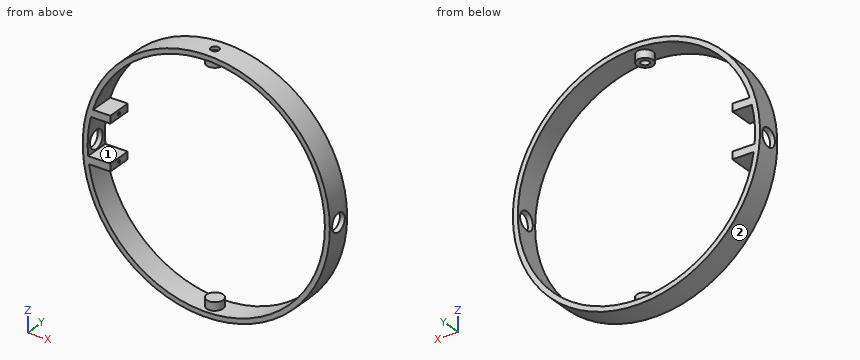
from build123d import *

# Parameters (mm, degrees)
SKETCH1_R               = 75
SKETCH1_R_2             = 72
BOSS_EXTRUDE1_DEPTH     = 15
SKETCH2_R               = 5.5
CUT_EXTRUDE1_DEPTH      = 76
CUT_EXTRUDE1_DEPTH_BACK = 76
BOSS_EXTRUDE2_START     = -6
SKETCH3_R               = 5
BOSS_EXTRUDE2_DEPTH     = 7
SKETCH4_W               = 11.8125703
SKETCH4_H               = 4.5
SKETCH4_W_2             = 13.541131856
BOSS_EXTRUDE3_DEPTH     = 15
SKETCH5_R               = 0.9
CUT_EXTRUDE2_DEPTH      = 8
SKETCH6_R               = 2.45
CUT_EXTRUDE3_DEPTH      = 4
SKETCH7_R               = 1.25
CUT_EXTRUDE4_DEPTH      = 4
SKETCH8_R               = 2.5
CUT_EXTRUDE5_DEPTH      = 4


with BuildPart() as part:
    # Sketch1 → Boss-Extrude1 (new body)
    with BuildSketch(Plane(origin=(0, 0, 0), x_dir=(1, 0, 0), z_dir=(0, 1, 0))):
        Circle(SKETCH1_R)
        Circle(SKETCH1_R_2, mode=Mode.SUBTRACT)
    extrude(amount=BOSS_EXTRUDE1_DEPTH)

    # Sketch2 → Cut-Extrude1 (cut, two sides)
    with BuildSketch(Plane(origin=(0, 0, 0), x_dir=(0, 0, -1), z_dir=(1, 0, 0))) as cut_extrude1_sk:
        with Locations((0, 7.5)):
            Circle(SKETCH2_R)
    extrude(amount=CUT_EXTRUDE1_DEPTH, mode=Mode.SUBTRACT)
    extrude(cut_extrude1_sk.sketch, amount=-CUT_EXTRUDE1_DEPTH_BACK, mode=Mode.SUBTRACT)

    # Sketch3 → Boss-Extrude2 (add)
    with BuildSketch(Plane.XY.offset(73).offset(BOSS_EXTRUDE2_START)):
        with Locations((0, 7.5)):
            Circle(SKETCH3_R)
    boss_extrude2 = extrude(amount=BOSS_EXTRUDE2_DEPTH)

    # Mirror1: Boss-Extrude2 across plane
    add(boss_extrude2.mirror(Plane.XY))

    # Sketch4 → Boss-Extrude3 (add)
    with BuildSketch(Plane(origin=(0, 15, 0), x_dir=(1, 0, 0), z_dir=(0, 1, 0))):
        with Locations((-64.10628515, -19.05)):
            Rectangle(SKETCH4_W, SKETCH4_H)
        with Locations((-64.970565928, 8.35)):
            Rectangle(SKETCH4_W_2, SKETCH4_H)
    extrude(amount=-BOSS_EXTRUDE3_DEPTH)

    # Sketch5 → Cut-Extrude2 (cut)
    with BuildSketch(Plane(origin=(-58.2, 0, 0), x_dir=(0, 0, -1), z_dir=(1, 0, 0))):
        with Locations((8.3, 7.5)):
            Circle(SKETCH5_R)
        with Locations((-19, 7.5)):
            Circle(SKETCH5_R)
    extrude(amount=-CUT_EXTRUDE2_DEPTH, mode=Mode.SUBTRACT)

    # Sketch6 → Cut-Extrude3 (cut)
    with BuildSketch(Plane(origin=(0, 0, 67), x_dir=(-1, 0, 0), z_dir=(0, 0, -1))):
        with Locations((0, 7.5)):
            Circle(SKETCH6_R)
    extrude(amount=-CUT_EXTRUDE3_DEPTH, mode=Mode.SUBTRACT)

    # Sketch7 → Cut-Extrude4 (cut)
    with BuildSketch(Plane(origin=(0, 0, 71), x_dir=(-1, 0, 0), z_dir=(0, 0, -1))):
        with Locations((0, 7.5)):
            Circle(SKETCH7_R)
    extrude(amount=-CUT_EXTRUDE4_DEPTH, mode=Mode.SUBTRACT)

    # Sketch8 → Cut-Extrude5 (cut)
    with BuildSketch(Plane(origin=(0, 0, 73), x_dir=(-1, 0, 0), z_dir=(0, 0, -1))):
        with Locations((0, 7.5)):
            Circle(SKETCH8_R)
    extrude(amount=-CUT_EXTRUDE5_DEPTH, mode=Mode.SUBTRACT)


solid = part.part
Source: CAD feature listing. Evaluate the final solid. Frame: model axes, mm. Face numbers are marked on the shaded views. Round coordinates to 2 decimals unless told otherwise and drop trailing zeros. Write each loop counter-clockwise with the first axis right and the second up, starting at its lowest first coordinate (ties: lowest second). Pieces come first, ordered by that corner, then holes. Notation, with made-up numbers: M -38.75,-28.5 L -28.75,-28.5 A21 cw -28.75,-8.5 Z; hole C 86.25,-29 d5. An arc over 180 degrees is marked long. One line per item, written item: value. Start each with the question number.
Item 1: Ray query, L1, parallel to Y at x = 0, z = 69; L2, parallel to Y at x = -73.8, z = 0; L3, parallel to Z at x = -63.5, y = 14.25. Return the intervals inside material, ascending. Write a range as from..to.
Item 2: Mould query, pull axis Z, two halves, no side actions, for the marked faces 1 and 2. Classes: pulls with the +Z half, pulls with the -Z half, needs draft (parallel to the pull), parting line crosses it, or undercut.
Item 3: Section query A-A (z = -13). Return the cut outline in (x, y), plus the area to 3 significant figures.
Item 4: Pin query (flat end, axial travel): pin 1 (1.5 mm diameter, centred on x = -54, y = 12, fed in from +Z); pin 2 (1.4 mm diameter, centred on y = 7.5, z = -8.3, fed in from +X); pin 3 (4 mm diameter, centred on x = 0, y = 7.5, fed in from +Z). Return the tip coordinate at first contact, or that it passes through.
Item 5: Section query B-B (x = 25). Return the cut outline in (y, z).
Result set:
1. L1: y = 2.5..5.05, 9.95..12.5
1. L2: y = 0..2, 13..15
1. L3: z = -39.91..-33.94, -10.6..-6.1, 16.8..21.3, 33.94..39.91
2. face 1: undercut
2. face 2: parting line crosses it
3. outline: M -73.86,0 L -70.82,0 L -70.82,15 L -73.86,15 Z; M 70.82,0 L 73.86,0 L 73.86,15 L 70.82,15 Z
3. area: 91.4 mm²
4. pin 1: stops at z = 52.82
4. pin 2: stops at x = 74.61
4. pin 3: stops at z = 73
5. outline: M 0,-70.71 L 15,-70.71 L 15,-67.52 L 0,-67.52 Z; M 0,67.52 L 15,67.52 L 15,70.71 L 0,70.71 Z
